Autodesk Inventor part; units mm, degrees
ref_plane "YZ Plane" through (0, 0, 0) normal (1, 0, 0) x (0, 1, 0)
ref_plane "XZ Plane" through (0, 0, 0) normal (0, 1, 0) x (-1, 0, 0)
ref_plane "XY Plane" through (0, 0, 0) normal (0, 0, 1) x (1, 0, 0)
sketch "Skizze1" plane through (0, 0, 0) normal (1, 0, 0) x (0, 1, 0)
  line L0 (-50, 36.5) -> (50, 36.5)
  line L1 (50, 36.5) -> (50, -36.5)
  line L2 (50, -36.5) -> (-50, -36.5)
  line L3 (-50, -36.5) -> (-50, 36.5)
  line L4 (-50, 36.5) -> (50, -36.5) construction
  line L5 (50, 36.5) -> (-50, -36.5) construction
  point P0 (0, 0)
  dimension "d0" = 73
  dimension "d1" = 100
extrude "Extrusion1" add sketch "Skizze1" along normal blind 5
chamfer "Fase1" distance 5 angle 45 1 edges at (5, 50, 0)
sketch "Skizze2" plane through (5, 0, 0) normal (1, 0, 0) x (0, 0, -1)
  line L0 (-36.5, 45) -> (-36.5, -50)
  line L1 (-36.5, 45) -> (36.5, 45)
  line L2 (-36.5, -50) -> (36.5, -50)
  line L3 (0, -70) -> (0, 70) construction
  point P0 (0, 0)
  point P1 (-31.5, -45)
  point P2 (-31.5, 40)
  point P3 (31.5, -45)
  point P4 (31.5, 40)
  dimension "d7" = 5
  dimension "d8" = 5
  dimension "d9" = 5
  dimension "d10" = 5
hole "Bohrung1" at (5, -45, 31.5) at (5, 40, 31.5) at (5, 40, -31.5) at (5, -45, -31.5) direction (-1, 0, 0) diameter 4 end through all counterbore diameter 7 counterbore depth 2
properties part number "Deckel_2_Frame" material "PC/ABS-Kunststoff"
Model file for the job. Use its own axes, mm. A direction names the side the tool comes from. Round coordinates to 2 decimals unless told otherwise and drop trailing zeros. Order: outer loops, then holes, each group sorted by start corner. A loop starts at its lowest first (then second) coordinate and runs counter-clockwise, first axis right, second up. Notation, with made-up numbers: M -14,12.25 L -6,12.25 A27 cw -6,32.25 Z; hole C 65.5,89 d5. An arc over 180 degrees is marked long. Write each question's results on one line, items separated by ' | '. Start each with the question number.
(1) Saw through at A-A, the plane y = -45. Give the cut face in (x, z), then the cut area to 3 significant figures.
(2) Probe probe 1 along Z at (x, y) = (0.9, 40); probe 2 along Z at (x, y) = (3.85, -45); probe 3 along Y at (x, z) = (4.4, 31.5). List the from-to ranges inside material, lowest first. Write a range as from..to.
(3) Drop flat-ended pins along their axis: pin 1 (11 mm diameter, centred on y = -45, z = -31.5, fed in from -X); pin 2 (2 mm diameter, centred on y = -44, z = 32, fed in from +X); pin 3 (2.5 mm diameter, centred on y = 40, z = -31.5, fed in from -X). Give the stop position or say it passes through.
(4) Which spindle directions (+Z, -Z, +X, -X, +Y, -Y) get a long thin tool onto all of the face, cutting with end or side? Do faces 4 (the face through (1.479, -43.226, -32.423)), 5 (the face through (3, -43, 30)). Say none if no direction does.
(5) Saw through at C-C, the plane x = 4.1. Give the cut face in (y, z).
(6) Saw through at B-B, the plane z = -31.5. State how many separate pieces and enclosed holes the cut face has, then the cut area to 3 significant figures.
(7) Two-plate mould, pull along Y, no slides. Class faces 1 (the face through (2, -1, 36.5)), 2 (the face through (1.479, -43.226, 30.577)), 3 (the face through (2, -50, -1)): pulls with the +Y half, pulls with the -Y half, needs draft (parallel to the pull), parting line crosses it, or undercut.
Established:
1) outline: M 0,-36.5 L 5,-36.5 L 5,-35 L 3,-35 L 3,-33.5 L 0,-33.5 Z; M 0,-29.5 L 3,-29.5 L 3,-28 L 5,-28 L 5,28 L 3,28 L 3,29.5 L 0,29.5 Z; M 0,33.5 L 3,33.5 L 3,35 L 5,35 L 5,36.5 L 0,36.5 Z | area: 313 mm^2
2) probe 1: z = -36.5..-33.5, -29.5..29.5, 33.5..36.5 | probe 2: z = -36.5..-35, -28..28, 35..36.5 | probe 3: y = -50..-48.5, -41.5..36.5, 43.5..45.6
3) pin 1: stops at x = 0 | pin 2: stops at x = 3 | pin 3: passes through
4) face 4: +X, -X | face 5: +X
5) outline: M -50,-36.5 L 45.9,-36.5 L 45.9,36.5 L -50,36.5 Z; hole C -45,-31.5 d7; hole C -45,31.5 d7; hole C 40,-31.5 d7; hole C 40,31.5 d7
6) separate pieces: 3 | enclosed holes: 0 | area: 436 mm^2
7) face 1: needs draft | face 2: undercut | face 3: pulls with the -Y half
